Here's how the part is built. I have some questions about the finished solid (model axes, mm). Face numbers are marked on the shaded views. Coordinates: 2 decimals unless noted, no trailing zeros. Order: outer loops, then holes, each group sorted by start corner. A loop starts at its lowest first (then second) coordinate and runs counter-clockwise, first axis right, second up. Notation, with made-up numbers: (42, 29.5) - (86, 29.5) arc R19 cw to (86, 52.5) - close; hole circle Ø8 at (-28, 71.25). An arc over 180 degrees is marked (long way). Answer as CSV lines item,"result". Start each with the question number.
Item 1: I'm going to push flat-ended pins straight in: pin 1 (1 mm diameter, centred on y = 13, z = 21.5, fed in from +X); pin 2 (3 mm diameter, centred on x = -1.5, y = 19.5, fed in from -Z); pin 3 (1.4 mm diameter, centred on x = -1.5, z = 22, fed in from +Y). Where does each tip first touch, or does it pass through?
Item 2: I need wall thicknesses on line 1 (Z direction, x = -1.55, y = 8.5); line 2 (Y direction, x = -0.6, z = 2.5); line 3 (Z direction, x = -4.9, y = 39). Which ranges of each line are inside material? Lowest first, please.
Item 3: Imagine slicing it at D-D on x = -0.85. Count the separate pieces of the cut face and the enclosed holes in it, and give its area (3 significant figures).
Item 4: Imagine slicing it at A-A on z = 14. List the corners of the cut face in (x, y) for me.
Item 5: Imagine slicing it at C-C on y = 23.5. List the corners of the cut face in (x, z) for me, and give its area (3 significant figures).
Item 6: We'd pull the mould along Z, two halves only. Please class the marked faces 1, 2, 3 and 4: pulls with the +Z half, pulls with the -Z half, needs draft (parallel to the pull), parting line crosses it, or undercut.
Item 7: Imagine slicing it at B-B on y = 40.5. List the corners of the cut face in (x, z) for me.
from build123d import *

# Parameters (mm, degrees)
BOSS_EXTRUDE1_DEPTH                   = 35.56
FILLET1_R                             = 12.7
SKETCH6_W                             = 24.384
SKETCH6_H                             = 44.958
CUT_EXTRUDE1_DEPTH                    = 2.794
FILLET2_R                             = 1.27
CUT_EXTRUDE3_DEPTH                    = 63.260576162
CUT_EXTRUDE4_DEPTH                    = 63.260576162
F_7_8_0_875_DIAMETER_HOLE1_D          = 22.225
F_40_0_098_DIAMETER_HOLE1_D           = 2.4892
F_40_0_098_DIAMETER_HOLE1_CSINK_D     = 3.7592
F_40_0_098_DIAMETER_HOLE1_CSINK_ANGLE = 90


with BuildPart() as part:
    # Sketch1 → Boss-Extrude1 (new body)
    with BuildSketch(Plane.XY):
        Polygon((0, 0), (0, 50.8), (-5.588, 50.8), (-5.588, 17.78), (-1.916643762, 0), align=None)
    extrude(amount=BOSS_EXTRUDE1_DEPTH)

    # Fillet1
    fillet1_edges = [part.edges().sort_by_distance(p)[0] for p in [
        (-5.588, 17.78, 17.78),
    ]]
    fillet(fillet1_edges, radius=FILLET1_R)

    # Sketch6 → Cut-Extrude1 (cut)
    with BuildSketch(Plane(origin=(0, 0, 0), x_dir=(0, 0, -1), z_dir=(1, 0, 0))):
        with Locations((-17.580042727, 28.321)):
            Rectangle(SKETCH6_W, SKETCH6_H)
    extrude(amount=-CUT_EXTRUDE1_DEPTH, mode=Mode.SUBTRACT)

    # Fillet2
    fillet2_edges = [part.edges().sort_by_distance(p)[0] for p in [
        (-1.397, 5.842, 29.772042727),
        (-1.397, 5.842, 5.388042727),
    ]]
    fillet(fillet2_edges, radius=FILLET2_R)

    # Sketch10 → Cut-Extrude3 (cut, through all)
    with BuildSketch(Plane(origin=(0, 0, 0), x_dir=(0, 0, -1), z_dir=(1, 0, 0))):
        Polygon((-35.56, 44.780420684), (-30.397580851, 50.8), (-35.56, 50.8), align=None)
    extrude(amount=-CUT_EXTRUDE3_DEPTH, mode=Mode.SUBTRACT)

    # Sketch11 → Cut-Extrude4 (cut, through all)
    with BuildSketch(Plane(origin=(0, 0, 0), x_dir=(0, 0, -1), z_dir=(1, 0, 0))):
        Polygon((-5.085545117, 50.8), (0, 50.8), (0, 44.824895363), align=None)
        Polygon((0, 6.029531172), (-5.128692816, 0), (0, 0), align=None)
        Polygon((-35.56, 6.07121688), (-35.56, 0), (-30.417091858, 0), align=None)
    extrude(amount=-CUT_EXTRUDE4_DEPTH, mode=Mode.SUBTRACT)

    # 7/8 (0.875) Diameter Hole1 (through all)
    with Locations(Plane.ZY.offset(5.588)):
        with Locations((17.678535919, 38.809523369)):
            Hole(F_7_8_0_875_DIAMETER_HOLE1_D / 2)

    # #40 (0.098) Diameter Hole1 (through all)
    with Locations(Plane.ZY.offset(5.588)):
        with Locations((2.678535919, 43.309523369), (2.678535919, 26.309523369), (2.678535919, 9.309523369), (9.178535919, 3.009523369), (26.181895158, 2.999179942), (32.672944692, 9.309523369), (32.678535919, 26.309523369), (32.678535919, 43.309523369)):
            CounterSinkHole(F_40_0_098_DIAMETER_HOLE1_D / 2, F_40_0_098_DIAMETER_HOLE1_CSINK_D / 2, counter_sink_angle=F_40_0_098_DIAMETER_HOLE1_CSINK_ANGLE)


solid = part.part
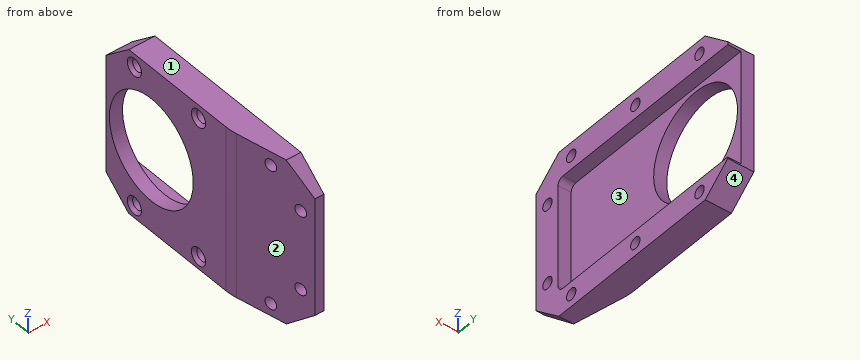
Responses:
1,pin 1,"stops at x = -2.79"
1,pin 2,"stops at z = 0"
1,pin 3,"stops at y = 5.84"
2,line 1,"z = 0 to 1.73, 3.62 to 5.39, 29.77 to 31.73, 33.62 to 35.56"
2,line 2,"y = 3.09 to 8.08, 10.54 to 25.08, 27.54 to 42.08, 44.54 to 47.76"
2,line 3,"z = 0 to 6.57, 28.79 to 35.56"
3,separate pieces,"1"
3,enclosed holes,"8"
3,area,"610 mm^2"
4,outline,"(-5.59, 19.08) arc R12.7 ccw to (-5.33, 16.51) - (-1.92, 0) - (0, 0) - (0, 5.84) - (-2.79, 5.84) - (-2.79, 28.32) - (-5.59, 28.32) - close; (-5.59, 49.3) - (-2.79, 49.3) - (-2.79, 50.8) - (-5.59, 50.8) - close"
5,outline,"(-5.59, 0) - (0, 0) - (0, 5.39) - (-2.79, 5.39) - (-2.79, 29.77) - (0, 29.77) - (0, 35.56) - (-5.59, 35.56) - close"
5,area,"131 mm^2"
6,face 1,"pulls with the +Z half"
6,face 2,"needs draft"
6,face 3,"undercut"
6,face 4,"pulls with the -Z half"
7,outline,"(-5.59, 0) - (0, 0) - (0, 5.39) - (-2.79, 5.39) - (-2.79, 6.7) - (-5.59, 6.7) - close; (-5.59, 28.66) - (-2.79, 28.66) - (-2.79, 29.77) - (0, 29.77) - (0, 35.56) - (-5.59, 35.56) - close"
